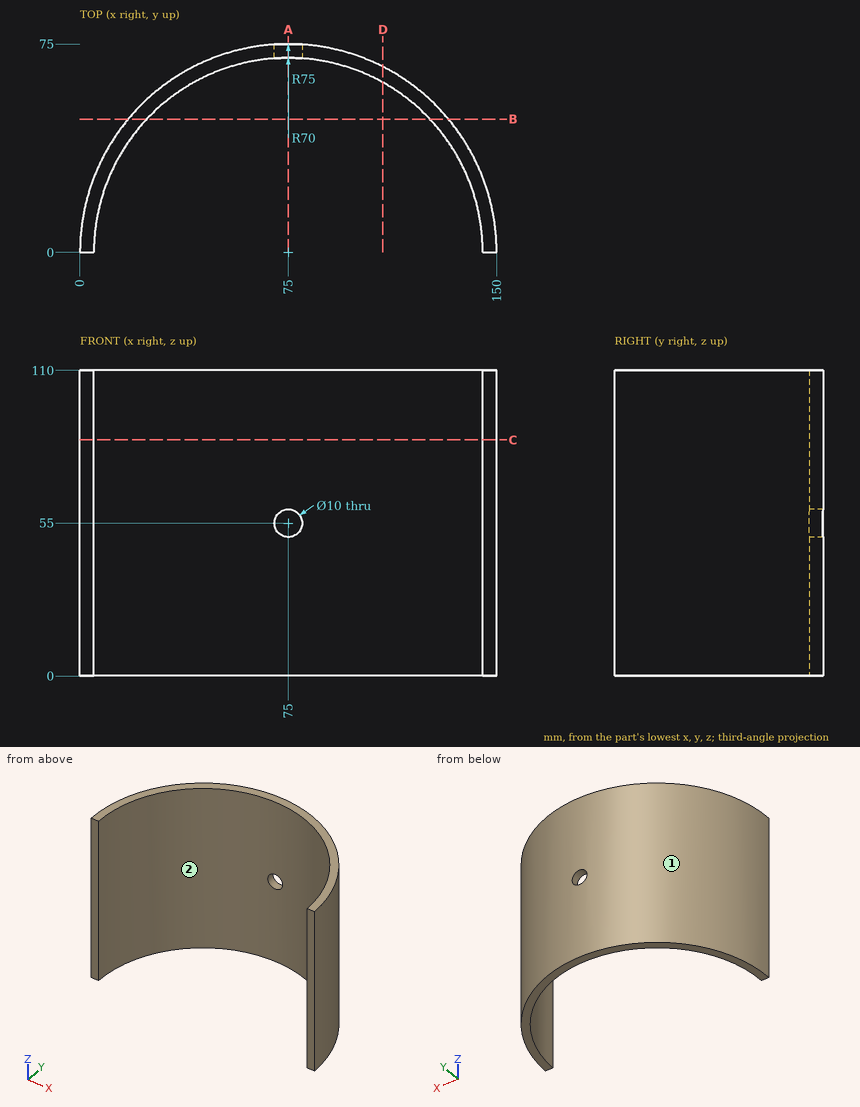
Answer from the drawing. Dimensions are ordinates in mm from the lowest x, y and z of the part. Round coordinates to 2 decimals unless told otherwise and drop trailing zeros. Write each loop counter-clockwise with the first axis right and the second up, starting at its lowest first coordinate (ties: lowest second). Pieces come first, ordered by that corner, then holes. Notation, with made-up numbers: (72.5, 55) - (77.5, 55) arc R18 cw to (77.5, 78) - close; hole circle Ø8 at (12.5, 14). An arc over 180 degrees is marked (long way). Use a Markdown table: item, result.
(1) Straight lines are drawn through the part: line 1 along Z through (x, y) = (75, 73); line 2 along X through (y, z) = (44, 45); line 3 along X through (y, z) = (27.5, 96). For each, find the intervals that lie inside material, in ascending order. Write a range as [from, to].
Reported:
| item | result |
|---|---|
| line 1 | [0, 50], [60, 110] |
| line 2 | [14.26, 20.56], [129.44, 135.74] |
| line 3 | [5.22, 10.63], [139.37, 144.78] |
(2) The part is cut by section C-C (z = 85). Write down the section's boundary in (x, y).
Reported:
| item | result |
|---|---|
| outline | (0, 0) - (5, 0) arc R70 cw to (145, 0) - (150, 0) arc R75 ccw to start |
(3) The part is cut by section D-D (x = 109). Write down the section's boundary in (y, z).
Reported:
| item | result |
|---|---|
| outline | (61.19, 0) - (66.85, 0) - (66.85, 110) - (61.19, 110) - close |
(4) Each of these flat-tipped pins is pushed along its axis until it touches: pin 1 Ø4 at (y, z) = (15, 46) entering from -X; pin 2 Ø5 at (y, z) = (54, 14.5) entering from -X; pin 3 Ø13 at (x, z) = (75, 55) entering from -Y. Where does it stop, or does it pass through?
Reported:
| item | result |
|---|---|
| pin 1 | x = 1.14 |
| pin 2 | x = 20.48 |
| pin 3 | y = 69.7 |
(5) The mould has two halves that part along X. Classify the marked faces 1 and 2: released by +X, released by -X, zero draft, split by the parting line, or undercut.
Reported:
| item | result |
|---|---|
| face 1 | split by the parting line |
| face 2 | undercut |
(6) The part is cut by section B-B (y = 48). Write down the section's boundary in (x, z).
Reported:
| item | result |
|---|---|
| outline | (17.37, 0) - (24.05, 0) - (24.05, 110) - (17.37, 110) - close; (125.95, 0) - (132.63, 0) - (132.63, 110) - (125.95, 110) - close |
(7) The part is cut by section A-A (x = 75). Write down the section's boundary in (y, z).
Reported:
| item | result |
|---|---|
| outline | (70, 0) - (75, 0) - (75, 50) - (70, 50) - close; (70, 60) - (75, 60) - (75, 110) - (70, 110) - close |
